```python
from build123d import *

# Parameters (mm, degrees)
F0_R         = 5
F1_DEPTH     = 10
F2_R         = 7.5
F2_R_2       = 5
F3_DEPTH     = 15
F5_DEPTH     = 5
F6_T1_DEPTH  = 16.216012475
F6_T6_ANGLE  = 57.151354628
F6_T11_ANGLE = 114.30679143
F6_T17_ANGLE = 57.151354628
F6_T23_ANGLE = 57.151354628
F6_T27_DEPTH = 27.4320249501
F6_T34_DEPTH = 27.4320249501
F6_T38_ANGLE = 114.30679143
F6_T45_ANGLE = 114.30679143
F6_T49_DEPTH = 27.4320249501
F6_T56_DEPTH = 27.4320249501
F6_T60_ANGLE = 57.151354628
F7_R         = 2
F8_DEPTH     = 5
F9_W         = 6.5028829414
F9_H         = 5
F10_DEPTH    = 6
F11_R        = 1


# Not quite as in the source:
# - a fillet or chamfer that OpenCascade refuses, or shapes differently, is made with other operations: its cross-section is extruded or revolved along the edge and cut away or added


with BuildPart() as f1:
    # F0 (on Top) → F1 (new body)
    with BuildSketch(Plane.XY):
        Circle(F0_R)
    extrude(amount=F1_DEPTH)

    # F2 (on face) → F3 (join)
    with BuildSketch(Plane.XY.offset(10)):
        Circle(F2_R)
        Circle(F2_R_2, mode=Mode.SUBTRACT)
        Circle(F2_R_2)
    extrude(amount=F3_DEPTH)

    # F4 (on face) → F5 (cut)
    with BuildSketch(Plane.XY.offset(25)):
        with BuildLine():
            Line((-10.1172067225, -2.4360036477), (-7.0933691733, -2.4360036477))
            ThreePointArc((-7.0933691733, -2.4360036477), (-7.5, 0), (-7.0933691733, 2.4360036477))
            Line((-7.0933691733, 2.4360036477), (-10.1172067225, 2.4360036477))
            Line((-10.1172067225, 2.4360036477), (-10.1172067225, -2.4360036477))
        make_face()
        with BuildLine():
            Line((-7.0933691733, -2.4360036477), (7.0933691733, -2.4360036477))
            ThreePointArc((7.0933691733, -2.4360036477), (7.3976438411, -1.2348544855), (7.5, 0))
            ThreePointArc((7.5, 0), (7.3976438411, 1.2348544855), (7.0933691733, 2.4360036477))
            Line((7.0933691733, 2.4360036477), (-7.0933691733, 2.4360036477))
            ThreePointArc((-7.0933691733, 2.4360036477), (-7.5, 0), (-7.0933691733, -2.4360036477))
        make_face()
        with BuildLine():
            Line((7.0933691733, -2.4360036477), (10.1172067225, -2.4360036477))
            Line((10.1172067225, -2.4360036477), (10.1172067225, 2.4360036477))
            Line((10.1172067225, 2.4360036477), (7.0933691733, 2.4360036477))
            ThreePointArc((7.0933691733, 2.4360036477), (7.3976438411, 1.2348544855), (7.5, 0))
            ThreePointArc((7.5, 0), (7.3976438411, -1.2348544855), (7.0933691733, -2.4360036477))
        make_face()
    extrude(amount=-F5_DEPTH, mode=Mode.SUBTRACT)

    # F6: fillet of radius 2 on 7 edges, made by hand

    # F6_s2 → F6_t1 (cut)
    with BuildSketch(Plane.XY.offset(20)):
        with BuildLine():
            ThreePointArc((-4.4337838236, 6.0490958833), (-5.1522550427, 3.8139845448), (-3.2514414707, 2.4360036477))
            Line((-3.2514414707, 2.4360036477), (-7.0933691733, 2.4360036477))
            ThreePointArc((-7.0933691733, 2.4360036477), (-6.0400681229, 4.4460743438), (-4.4337838236, 6.0490958833))
        make_face()
        with BuildLine():
            ThreePointArc((4.4337838236, 6.0490958833), (5.1522550427, 3.8139845448), (3.2514414707, 2.4360036477))
            Line((3.2514414707, 2.4360036477), (7.0933691733, 2.4360036477))
            ThreePointArc((7.0933691733, 2.4360036477), (6.0400681229, 4.4460743438), (4.4337838236, 6.0490958833))
        make_face()
        with BuildLine():
            ThreePointArc((4.4337838236, -6.0490958833), (5.1522550427, -3.8139845448), (3.2514414707, -2.4360036477))
            Line((3.2514414707, -2.4360036477), (7.0933691733, -2.4360036477))
            ThreePointArc((7.0933691733, -2.4360036477), (6.0400681229, -4.4460743438), (4.4337838236, -6.0490958833))
        make_face()
        with BuildLine():
            ThreePointArc((-4.4337838236, -6.0490958833), (-5.1522550427, -3.8139845448), (-3.2514414707, -2.4360036477))
            Line((-3.2514414707, -2.4360036477), (-7.0933691733, -2.4360036477))
            ThreePointArc((-7.0933691733, -2.4360036477), (-6.0400681229, -4.4460743438), (-4.4337838236, -6.0490958833))
        make_face()
    extrude(amount=F6_T1_DEPTH, mode=Mode.SUBTRACT)


with BuildPart() as f6_tool4:
    # F6_s5 → F6_t6 (revolve)
    with BuildSketch(Plane.XZ):
        with BuildLine():
            ThreePointArc((7.5, 18), (6.9142135624, 19.4142135624), (5.5, 20))
            Line((5.5, 20), (7.5, 20))
            Line((7.5, 20), (7.5, 18))
        make_face()
    revolve(axis=Axis((0, 0, 20), (0, 0, -1)), revolution_arc=F6_T6_ANGLE)

    split(bisect_by=Plane.XZ.offset(2.4360036477), keep=Keep.BOTTOM)


with BuildPart() as f1_1:
    add(f1.part)

    # F6_t3: cut F6_tool4
    add(f6_tool4.part, mode=Mode.SUBTRACT)


with BuildPart() as f6_tool9:
    # F6_s10 → F6_t11 (revolve)
    with BuildSketch(Plane(origin=(0, 0, 0), x_dir=(0, 0, 1), z_dir=(0.840125701, -0.5423917464, 0))):
        with BuildLine():
            ThreePointArc((18, 7.5), (19.4142135624, 6.9142135624), (20, 5.5))
            Line((20, 5.5), (20, 7.5))
            Line((20, 7.5), (18, 7.5))
        make_face()
    revolve(axis=Axis((0, 0, 20), (0, 0, -1)), revolution_arc=F6_T11_ANGLE)

    split(bisect_by=Plane.XZ.offset(-2.4360036477), keep=Keep.TOP)

    split(bisect_by=Plane.XZ.offset(2.4360036477), keep=Keep.BOTTOM)


with BuildPart() as f1_2:
    add(f1_1.part)

    # F6_t8: cut F6_tool9
    add(f6_tool9.part, mode=Mode.SUBTRACT)


with BuildPart() as f6_tool15:
    # F6_s16 → F6_t17 (revolve)
    with BuildSketch(Plane(origin=(0, 0, 0), x_dir=(0, 0, 1), z_dir=(-0.8401063785, 0.5424216744, 0))):
        with BuildLine():
            ThreePointArc((18, 7.5), (19.4142135624, 6.9142135624), (20, 5.5))
            Line((20, 5.5), (20, 7.5))
            Line((20, 7.5), (18, 7.5))
        make_face()
    revolve(axis=Axis((0, 0, 20), (0, 0, -1)), revolution_arc=F6_T17_ANGLE)

    split(bisect_by=Plane.XZ.offset(-2.4360036477), keep=Keep.TOP)


with BuildPart() as f1_3:
    add(f1_2.part)

    # F6_t14: cut F6_tool15
    add(f6_tool15.part, mode=Mode.SUBTRACT)


with BuildPart() as f6_tool21:
    # F6_s22 → F6_t23 (revolve)
    with BuildSketch(Plane.XZ):
        with BuildLine():
            ThreePointArc((7.5, 18), (6.9142135624, 19.4142135624), (5.5, 20))
            Line((5.5, 20), (7.5, 20))
            Line((7.5, 20), (7.5, 18))
        make_face()
    revolve(axis=Axis((0, 0, 20), (0, 0, -1)), revolution_arc=F6_T23_ANGLE)

    split(bisect_by=Plane.XZ.offset(2.4360036477), keep=Keep.TOP)


with BuildPart() as f6_tool25:
    # F6_s26 → F6_t27 (new body)
    with BuildSketch(Plane.XY.offset(36.216012475)):
        with BuildLine():
            ThreePointArc((4.4337838236, -6.0490958833), (5.1522550427, -3.8139845448), (3.2514414707, -2.4360036477))
            Line((3.2514414707, -2.4360036477), (7.0933691733, -2.4360036477))
            ThreePointArc((7.0933691733, -2.4360036477), (6.0400681229, -4.4460743438), (4.4337838236, -6.0490958833))
        make_face()
    extrude(amount=-F6_T27_DEPTH)

    split(bisect_by=Plane.XY.offset(20), keep=Keep.BOTTOM)


with BuildPart() as f6_tool21_1:
    add(f6_tool21.part)

    # F6_t29: intersect F6_tool25
    add(f6_tool25.part, mode=Mode.INTERSECT)


with BuildPart() as f1_4:
    add(f1_3.part)

    # F6_t19: cut F6_tool21
    add(f6_tool21_1.part, mode=Mode.SUBTRACT)


with BuildPart() as f6_tool32:
    # F6_s33 → F6_t34 (new body)
    with BuildSketch(Plane.XY.offset(36.216012475)):
        with BuildLine():
            ThreePointArc((-4.4337838236, -6.0490958833), (-5.1522550427, -3.8139845448), (-3.2514414707, -2.4360036477))
            Line((-3.2514414707, -2.4360036477), (-7.0933691733, -2.4360036477))
            ThreePointArc((-7.0933691733, -2.4360036477), (-6.0400681229, -4.4460743438), (-4.4337838236, -6.0490958833))
        make_face()
    extrude(amount=-F6_T34_DEPTH)

    split(bisect_by=Plane.XY.offset(20), keep=Keep.BOTTOM)


with BuildPart() as f6_tool36:
    # F6_s37 → F6_t38 (revolve)
    with BuildSketch(Plane(origin=(0, 0, 0), x_dir=(0, 0, 1), z_dir=(0.840125701, -0.5423917464, 0))):
        with BuildLine():
            ThreePointArc((18, 7.5), (19.4142135624, 6.9142135624), (20, 5.5))
            Line((20, 5.5), (20, 7.5))
            Line((20, 7.5), (18, 7.5))
        make_face()
    revolve(axis=Axis((0, 0, 20), (0, 0, -1)), revolution_arc=F6_T38_ANGLE)

    split(bisect_by=Plane.XZ.offset(2.4360036477), keep=Keep.TOP)


with BuildPart() as f6_tool32_1:
    add(f6_tool32.part)

    # F6_t40: intersect F6_tool36
    add(f6_tool36.part, mode=Mode.INTERSECT)


with BuildPart() as f1_5:
    add(f1_4.part)

    # F6_t30: cut F6_tool32
    add(f6_tool32_1.part, mode=Mode.SUBTRACT)


with BuildPart() as f6_tool43:
    # F6_s44 → F6_t45 (revolve)
    with BuildSketch(Plane(origin=(0, 0, 0), x_dir=(0, 0, 1), z_dir=(0.840125701, -0.5423917464, 0))):
        with BuildLine():
            ThreePointArc((18, 7.5), (19.4142135624, 6.9142135624), (20, 5.5))
            Line((20, 5.5), (20, 7.5))
            Line((20, 7.5), (18, 7.5))
        make_face()
    revolve(axis=Axis((0, 0, 20), (0, 0, -1)), revolution_arc=F6_T45_ANGLE)

    split(bisect_by=Plane.XZ.offset(-2.4360036477), keep=Keep.BOTTOM)


with BuildPart() as f6_tool47:
    # F6_s48 → F6_t49 (new body)
    with BuildSketch(Plane.XY.offset(36.216012475)):
        with BuildLine():
            ThreePointArc((-4.4337838236, 6.0490958833), (-5.1522550427, 3.8139845448), (-3.2514414707, 2.4360036477))
            Line((-3.2514414707, 2.4360036477), (-7.0933691733, 2.4360036477))
            ThreePointArc((-7.0933691733, 2.4360036477), (-6.0400681229, 4.4460743438), (-4.4337838236, 6.0490958833))
        make_face()
    extrude(amount=-F6_T49_DEPTH)

    split(bisect_by=Plane.XY.offset(20), keep=Keep.BOTTOM)


with BuildPart() as f6_tool43_1:
    add(f6_tool43.part)

    # F6_t51: intersect F6_tool47
    add(f6_tool47.part, mode=Mode.INTERSECT)


with BuildPart() as f1_6:
    add(f1_5.part)

    # F6_t41: cut F6_tool43
    add(f6_tool43_1.part, mode=Mode.SUBTRACT)


with BuildPart() as f6_tool54:
    # F6_s55 → F6_t56 (new body)
    with BuildSketch(Plane.XY.offset(36.216012475)):
        with BuildLine():
            ThreePointArc((4.4337838236, 6.0490958833), (5.1522550427, 3.8139845448), (3.2514414707, 2.4360036477))
            Line((3.2514414707, 2.4360036477), (7.0933691733, 2.4360036477))
            ThreePointArc((7.0933691733, 2.4360036477), (6.0400681229, 4.4460743438), (4.4337838236, 6.0490958833))
        make_face()
    extrude(amount=-F6_T56_DEPTH)

    split(bisect_by=Plane.XY.offset(20), keep=Keep.BOTTOM)


with BuildPart() as f6_tool58:
    # F6_s59 → F6_t60 (revolve)
    with BuildSketch(Plane(origin=(0, 0, 0), x_dir=(0, 0, 1), z_dir=(-0.8401063785, 0.5424216744, 0))):
        with BuildLine():
            ThreePointArc((18, 7.5), (19.4142135624, 6.9142135624), (20, 5.5))
            Line((20, 5.5), (20, 7.5))
            Line((20, 7.5), (18, 7.5))
        make_face()
    revolve(axis=Axis((0, 0, 20), (0, 0, -1)), revolution_arc=F6_T60_ANGLE)

    split(bisect_by=Plane.XZ.offset(-2.4360036477), keep=Keep.BOTTOM)


with BuildPart() as f6_tool54_1:
    add(f6_tool54.part)

    # F6_t62: intersect F6_tool58
    add(f6_tool58.part, mode=Mode.INTERSECT)


with BuildPart() as f1_7:
    add(f1_6.part)

    # F6_t52: cut F6_tool54
    add(f6_tool54_1.part, mode=Mode.SUBTRACT)

    # F7
    f7_edges = [f1_7.edges().sort_by_distance(p)[0] for p in [
        (-5, 0, 0),
    ]]
    fillet(f7_edges, radius=F7_R)

    # F8 (add): faces of the model
    f8_faces = [f1_7.faces().sort_by_distance(p)[0] for p in [
        (0, 4.7439045523, 25),
        (0, -4.7439045523, 25),
    ]]
    extrude(f8_faces, amount=F8_DEPTH)

    # F9 (on face) → F10 (join)
    with BuildSketch(Plane.XZ.offset(-2.4360036477)):
        with Locations((0, 27.5)):
            Rectangle(F9_W, F9_H)
    extrude(amount=F10_DEPTH)

    # F11
    f11_edges = [f1_7.edges().sort_by_distance(p)[0] for p in [
        (3.251441, 0, 25),
        (-3.251441, 0, 25),
    ]]
    fillet(f11_edges, radius=F11_R)


solid = f1_7.part
```
Geometry: final body of the model. Coordinates: model frame, mm. A direction names the side the tool comes from. Coordinates: 2 decimals unless noted, no trailing zeros. Order: outer loops, then holes, each group sorted by start corner. A loop starts at its lowest first (then second) coordinate and runs counter-clockwise, first axis right, second up. Notation, with made-up numbers: (64, 85) -> (91, 85) arc R34 ccw to (91, 120) -> close; hole circle Ø8 at (10, 33). An arc over 180 degrees is marked (long way). Use CSV: the item, a comma, the result in double quotes.
1) Pin query (flat end, axial travel): pin 1 Ø2 at (y, z) = (-1, 28.5) entering from +X; pin 2 Ø3 at (x, z) = (0.5, 23) entering from -Y; pin 3 Ø1.5 at (y, z) = (3.5, 14) entering from +X; pin 4 Ø3 at (x, y) = (-3, -3.5) entering from -Z. Return the tip coordinate at first contact, or that it passes through.
Findings:
pin 1,"stops at x = 3.25"
pin 2,"stops at y = -7.5"
pin 3,"stops at x = 6.98"
pin 4,"stops at z = 0"
2) Section D-D on z = 9.5. Output: boundary loops of the cut face in (x, y), then the cut area to 3 significant figures.
Findings:
outline,"circle Ø10 at (0, 0)"
area,"78.5 mm^2"
3) Mould query, pull axis Z, two halves, no side actions, for faces 5 (the cylindrical face through (-5.14, 3.78, 25.25)), 6 (the flat face through (2, -5, 10)), 7 (the cylindrical face through (-2.966, -0.034, 25.301)). Classes: +Z half, -Z half, draft (parallel to the pull), parting line (faces both ways), or undercut.
Findings:
face 5,"draft"
face 6,"-Z half"
face 7,"undercut"
4) Section B-B on x = 0. Output: boundary loops of the cut face in (y, z).
Findings:
outline,"(-7.5, 10) -> (-5, 10) -> (-5, 2) arc R2 ccw to (-3, 0) -> (3, 0) arc R2 ccw to (5, 2) -> (5, 10) -> (7.5, 10) -> (7.5, 30) -> (-7.5, 30) -> close; hole (-2.44, 20) -> (2.44, 20) -> (2.44, 25) -> (-2.44, 25) -> close"
5) Line query: line 1 (Z direction, x = 0.5, y = 5.75); line 2 (X direction, y = -4.5, z = 21.5); line 3 (Z direction, x = -2.25, y = -0.25). Output: solid intervals per line, ascending.
Findings:
line 1,"z = 10 to 30"
line 2,"x = -5.25 to 5.25"
line 3,"z = 0 to 20, 25 to 30"
6) Section C-C on y = 0. Output: boundary loops of the cut face in (x, z), then the cut area to 3 significant figures.
Findings:
outline,"(-7.5, 10) -> (-5, 10) -> (-5, 2) arc R2 ccw to (-3, 0) -> (3, 0) arc R2 ccw to (5, 2) -> (5, 10) -> (7.5, 10) -> (7.5, 18) arc R2 ccw to (5.5, 20) -> (-5.5, 20) arc R2 ccw to (-7.5, 18) -> close; (-3.25, 26) arc R1 ccw to (-2.25, 25) -> (2.25, 25) arc R1 ccw to (3.25, 26) -> (3.25, 30) -> (-3.25, 30) -> close"
area,"279 mm^2"
7) Section A-A on z = 22. Output: boundary loops of the cut face in (x, y).
Findings:
outline,"(-4.43, -6.05) arc R7.5 ccw to (4.43, -6.05) arc R2 ccw to (3.25, -2.44) -> (-3.25, -2.44) arc R2 ccw to start; (-4.43, 6.05) arc R2 ccw to (-3.25, 2.44) -> (3.25, 2.44) arc R2 ccw to (4.43, 6.05) arc R7.5 ccw to start"
8) Access query for faces 1 (the flat face through (-3.251, 0, 28)), 2 (the cylindrical face through (2.951, -0.034, 25.285)), 3 (the flat face through (0, 0, 25)), 4 (the flat face through (3.251, 0, 28)). Directions: +Z, -Z, +X, -X, +Y, -Y. A direction counts if a zero-diameter tool reaches every point of the face in a straight line with its end or side. Return the directions, or none.
Findings:
face 1,"+Z, -X"
face 2,"+X"
face 3,"+X, -X"
face 4,"+Z, +X"
